Could you check a few things on this model? Use its own coordinates, in mm. Round coordinates to 2 decimals unless told otherwise and drop trailing zeros. Loops run counter-clockwise (first coordinate to the right, second up) from the corner with the lowest first, then second, coordinate; pieces in that order, holes last. Notation, with made-up numbers: (21, -1) -> (64, -1) arc R30 cw to (64, 33) -> close; hole circle Ø6 at (-38, 43.5). An arc over 180 degrees is marked (long way). Put each result on its own line as item: value. Start each with the question number.
1. I'm going to push flat-ended pins straight in: P1, Ø8, axis at x = -6, z = -12, coming from the +Y side; P2, Ø8, axis at x = -7.5, z = -6.5, coming from the +Y side; P3, Ø1.5, axis at x = -15.5, z = -11.5, coming from the -Y side. Where does each tip first touch, or does it pass through?
2. I need wall thicknesses on line 1 (Y direction, x = 0, z = -8.5); line 2 (Y direction, x = -5, z = -1.5); line 3 (X direction, y = 1, z = -12.5). Which ranges of each line are inside material? Lowest first, please. Write a range as [from, to].
3. Imagine slicing it at C-C, the plane z = -4. Please give me the cut outline in (x, y), and give its area (3 significant figures).
4. Imagine slicing it at A-A, the plane x = 0. Please give me the cut outline in (y, z), and give its area (3 significant figures).
5. If we mould it in two halves opening along X, with no side actions, what happens to faces 1 (the cylindrical face through (4.336, -19.524, -7.084)), 2 (the flat face through (-4.1, -18.2, 0)), 3 (the cylindrical face through (13.887, 10.648, -6.916))? For each: pulls with the +X half, pulls with the -X half, needs draft (parallel to the pull), parting line crosses it, or undercut.
Autodesk Inventor part; units mm, degrees
ref_plane "YZ Plane" through (0, 0, 0) normal (1, 0, 0) x (0, 1, 0)
ref_plane "XZ Plane" through (0, 0, 0) normal (0, 1, 0) x (-1, 0, 0)
ref_plane "XY Plane" through (0, 0, 0) normal (0, 0, 1) x (1, 0, 0)
sketch "Sketch1" plane through (0, 0, 0) normal (0, 1, 0) x (-1, 0, 0)
  line L0 (0, 0) -> (0, -14) construction
  line L1 (18.5, 0) -> (19, 0)
  line L2 (20, -1) -> (20, -13)
  line L3 (19, -14) -> (18.5, -14)
  line L4 (17.5, -13) -> (17.5, -1)
  arc A0 (20, -1) -> (19, 0) centre (19, -1) ccw
  arc A1 (19, -14) -> (20, -13) centre (19, -13) ccw
  line L5 (18.5, 0) -> (17.5, -1)
  line L6 (18.5, -14) -> (17.5, -13)
  dimension "d0" = 14
  dimension "d1" = 17.5
  dimension "d2" = 20
  dimension "d3" = 14
  dimension "d4" = 1
  dimension "d5" = 18.5
  dimension "d6" = 1
  dimension "d7" = 18.5
  dimension "d8" = 1
revolve "Revolution1" add sketch "Sketch1" angle 360 about axis through (0, 0, 0) along (0, 0, -1)
properties part number "26-10-206 Spannrad Stufe 2, Riemenspanner"
Entries:
1. P1: y = 19.9
1. P2: y = 19.69
1. P3: y = -13.51
2. line 1: [-20, -17.5], [17.5, 20]
2. line 2: [-19.36, -16.77], [16.77, 19.36]
2. line 3: [-19.97, -17.47], [17.47, 19.97]
3. outline: circle Ø40 at (0, 0); hole circle Ø35 at (0, 0)
3. area: 295 mm^2
4. outline: (-20, -13) arc R1 ccw to (-19, -14) -> (-18.5, -14) -> (-17.5, -13) -> (-17.5, -1) -> (-18.5, 0) -> (-19, 0) arc R1 ccw to (-20, -1) -> close; (17.5, -13) -> (18.5, -14) -> (19, -14) arc R1 ccw to (20, -13) -> (20, -1) arc R1 ccw to (19, 0) -> (18.5, 0) -> (17.5, -1) -> close
4. area: 67.1 mm^2
5. face 1: parting line crosses it
5. face 2: needs draft
5. face 3: undercut
